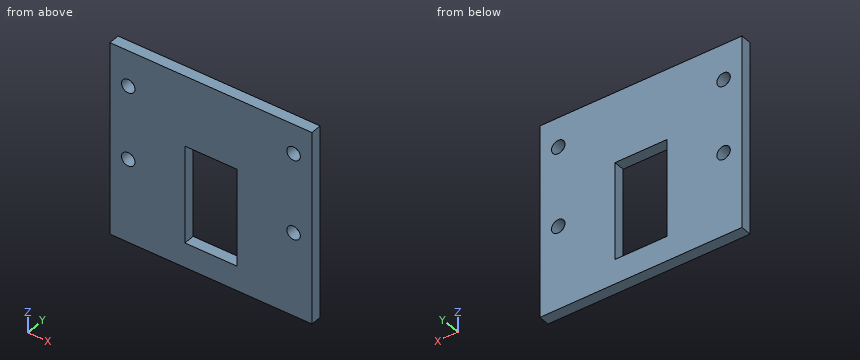
```python
from build123d import *

# Parameters (mm, degrees)
SKETCH5_W      = 41.91
SKETCH5_H      = 39.878
SKETCH5_R      = 1.397
EXTRUDE3_DEPTH = 2.286
SKETCH6_W      = 10.7696
SKETCH6_H      = 20.1676
EXTRUDE4_DEPTH = 3.286


with BuildPart() as part:
    # Sketch5 → Extrude3 (new body)
    with BuildSketch(Plane(origin=(0, 0, 0), x_dir=(1, 0, 0), z_dir=(0, 1, 0))):
        with Locations((-20.955, -19.939)):
            Rectangle(SKETCH5_W, SKETCH5_H)
        with Locations((-38.1, -17.272)):
            Circle(SKETCH5_R, mode=Mode.SUBTRACT)
        with Locations((-38.1, -32.512)):
            Circle(SKETCH5_R, mode=Mode.SUBTRACT)
        with Locations((-3.81, -33.782)):
            Circle(SKETCH5_R, mode=Mode.SUBTRACT)
        with Locations((-3.81, -17.272)):
            Circle(SKETCH5_R, mode=Mode.SUBTRACT)
    extrude(amount=EXTRUDE3_DEPTH)

    # Sketch6 → Extrude4 (cut, through all)
    with BuildSketch(Plane(origin=(0, 2.286, 0), x_dir=(-1, 0, 0), z_dir=(0, 1, 0))):
        with Locations((20.955, 15.1892)):
            Rectangle(SKETCH6_W, SKETCH6_H)
    extrude(amount=-EXTRUDE4_DEPTH, mode=Mode.SUBTRACT)


solid = part.part
```
Input: part model. Units: mm. Frame: model coordinates. Coordinates: 2 decimals unless noted, no trailing zeros. Order: outer loops, then holes, each group sorted by start corner. A loop starts at its lowest first (then second) coordinate and runs counter-clockwise, first axis right, second up. Notation, with made-up numbers: (32, -16) - (62, -16) arc R21 cw to (62, -11) - close; hole circle Ø6 at (-39, 36.25). An arc over 180 degrees is marked (long way). Put each result on its own line as item: value.
1. Cut plane C-C on y = 1.05. Return the cut outline in (x, z), then the cut area to 3 significant figures.
Report:
outline: (-41.91, 0) - (0, 0) - (0, 39.88) - (-41.91, 39.88) - close; hole circle Ø2.79 at (-38.1, 17.27); hole circle Ø2.79 at (-38.1, 32.51); hole (-26.34, 5.11) - (-15.57, 5.11) - (-15.57, 25.27) - (-26.34, 25.27) - close; hole circle Ø2.79 at (-3.81, 17.27); hole circle Ø2.79 at (-3.81, 33.78)
area: 1,430 mm2
2. Contact query for a flat-ended pin moving along its axis: pin 1 Ø1.7 at (x, z) = (-38.1, 17.272) entering from +Y. Output: stop coordinate, or through.
Report:
pin 1: passes through
3. Cut plane A-A on x = -38.1. Return the cut outline in (y, z) (3 decimals).
Report:
outline: (0, 0) - (2.286, 0) - (2.286, 15.875) - (0, 15.875) - close; (0, 18.669) - (2.286, 18.669) - (2.286, 31.115) - (0, 31.115) - close; (0, 33.909) - (2.286, 33.909) - (2.286, 39.878) - (0, 39.878) - close
4. Cut plane B-B on x = -21. Return the cut outline in (y, z).
Report:
outline: (0, 0) - (2.29, 0) - (2.29, 5.11) - (0, 5.11) - close; (0, 25.27) - (2.29, 25.27) - (2.29, 39.88) - (0, 39.88) - close
5. Line query: line 1 along Z through (x, y) = (-3.81, 0.55) (3 decimals); line 2 along X through (y, z) = (1.6, 23.5); line 3 along Z through (x, y) = (-3.5, 0.85). Output: solid intervals per line, ascending.
Report:
line 1: z = 0 to 15.875, 18.669 to 32.385, 35.179 to 39.878
line 2: x = -41.91 to -26.34, -15.57 to 0
line 3: z = 0 to 15.91, 18.63 to 32.42, 35.14 to 39.88
